Autodesk Inventor part; units mm, degrees
ref_plane "YZ Plane" through (0, 0, 0) normal (1, 0, 0) x (0, 1, 0)
ref_plane "XZ Plane" through (0, 0, 0) normal (0, 1, 0) x (-1, 0, 0)
ref_plane "XY Plane" through (0, 0, 0) normal (0, 0, 1) x (1, 0, 0)
sketch "Sketch1" plane through (0, 0, 0) normal (0, 1, 0) x (-1, 0, 0)
  circle A0 centre (0, 0) radius 13
  line L0 (-10.6616, 0) -> (-8.6254, 6.2667)
  line L1 (-8.6254, 6.2667) -> (-3.2946, 10.1398)
  line L2 (-3.2946, 10.1398) -> (3.2946, 10.1398)
  line L3 (3.2946, 10.1398) -> (8.6254, 6.2667)
  line L4 (8.6254, 6.2667) -> (10.6616, 0)
  line L5 (10.6616, 0) -> (8.6254, -6.2667)
  line L6 (8.6254, -6.2667) -> (3.2946, -10.1398)
  line L7 (3.2946, -10.1398) -> (-3.2946, -10.1398)
  line L8 (-3.2946, -10.1398) -> (-8.6254, -6.2667)
  line L9 (-8.6254, -6.2667) -> (-10.6616, 0)
  line L10 (-11.3, 0) -> (-9.1419, 6.642)
  line L11 (-9.1419, 6.642) -> (-3.4919, 10.7469)
  line L12 (-3.4919, 10.7469) -> (3.4919, 10.7469)
  line L13 (3.4919, 10.7469) -> (9.1419, 6.642)
  line L14 (9.1419, 6.642) -> (11.3, 0)
  line L15 (11.3, 0) -> (9.1419, -6.642)
  line L16 (9.1419, -6.642) -> (3.4919, -10.7469)
  line L17 (3.4919, -10.7469) -> (-3.4919, -10.7469)
  line L18 (-3.4919, -10.7469) -> (-9.1419, -6.642)
  line L19 (-9.1419, -6.642) -> (-11.3, 0)
  circle A1 centre (-6, 0) radius 3.75
  circle A2 centre (6, 0) radius 3.75
  line L20 (9.4432, -3.75) -> (-9.4432, -3.75)
  line L21 (-9.4432, 3.75) -> (9.4432, 3.75)
  dimension "d0" = 26
  dimension "d8" = 7.5
  dimension "d9" = 7.5
extrude "Extrusion1" add sketch "Sketch1" against normal blind 3 contours L10 L11 L12 L13 L14 L15 L16 L17 L18 L19
extrude "Extrusion2" add sketch "Sketch1" along normal blind 20 contours A0
extrude "Extrusion3" add sketch "Sketch1" along normal blind 15 contours L0 L1 L2 L3 L4 L21 | L20 L5 L6 L7 L8 L9 | L10 L11 L12 L13 L14 L15 L16 L17 L18 L19
properties part number "Probe P2"
Could you check a few things on this model? Use its own coordinates, in mm. A direction names the side the tool comes from. Give positions to 0.01 mm unless a question says otherwise; leave off trailing zeros. Order: outer loops, then holes, each group sorted by start corner. A loop starts at its lowest first (then second) coordinate and runs counter-clockwise, first axis right, second up. Notation, with made-up numbers: (67, 24.5) -> (122, 24.5) arc R13 ccw to (122, 43.5) -> close; hole circle Ø3 at (85, 1). An arc over 180 degrees is marked (long way). Answer in a Markdown table with one row per item. Add a question column.
Item 1: Imagine slicing it at D-D (z = -4.75). List the corners of the cut face in (x, y) for me, and give its area (3 significant figures).
Item 2: Imagine slicing it at C-C (y = -0.5). List the corners of the cut face in (x, z) for me, and give its area (3 significant figures).
Item 3: Please list where these lines run through material, in increasing order: probe 1 along Z at (x, y) = (-1.25, -0.75); probe 2 along Y at (x, z) = (-7, 6); probe 3 along X at (y, z) = (14.25, -1.5).
Item 4: I'm going to push flat-ended pins straight in: P1, Ø10, axis at x = 2, z = -2.5, coming from the -Y side; P2, Ø1, axis at y = 14.5, z = 8, coming from the +X side; P3, Ø1, axis at x = -2, y = 15.5, coming from the -Z side. Where does each tip first touch, or does it pass through?
Item 5: We'd pull the mould along X, two halves only. Please class faces 4 (the flat face through (-7, -3, -8)), 5 (the cylindrical face through (10.316, 9.86, 7.91)), 6 (the flat face through (10.236, 17.465, 3.275)), 7 (the flat face through (-6.356, -1.479, -8.666)): pulls with the +X half, pulls with the -X half, needs draft (parallel to the pull), parting line crosses it, or undercut.
Item 6: Imagine slicing it at B-B (z = 0.5). List the corners of the cut face in (x, y) for me, and give its area (3 significant figures).
Item 7: Imagine slicing it at A-A (x = 0). List the corners of the cut face in (y, z) for me.
Item 8: For faces 1 (the flat face through (-10.236, 17.465, -3.275)), 2 (the flat face through (6.28, -1.48, -8.72)), 3 (the flat face through (-5.997, -1.479, -8.176)), which set-ups out of +Z, -Z, +X, -X, +Y, -Y let a thin tool reach every point of the face, with its end or its side?
Result:
| question | item | result |
|---|---|---|
| 1 | outline | (-12.1, 0) -> (-9.76, 0) -> (-9.76, -3) -> (-9.12, -3) -> (-9.12, 0) -> (9.12, 0) -> (9.12, -3) -> (9.76, -3) -> (9.76, 0) -> (12.1, 0) -> (12.1, 20) -> (9.76, 20) -> (9.76, 15) -> (-9.76, 15) -> (-9.76, 20) -> (-12.1, 20) -> close |
| 1 | area | 390 mm2 |
| 2 | outline | (-11.3, 0) -> (-9.14, -6.64) -> (-3.49, -10.75) -> (3.49, -10.75) -> (9.14, -6.64) -> (11.3, 0) -> (9.14, 6.64) -> (3.49, 10.75) -> (-3.49, 10.75) -> (-9.14, 6.64) -> close; hole (-10.66, 0) -> (-8.63, -6.27) -> (-3.29, -10.14) -> (3.29, -10.14) -> (8.63, -6.27) -> (10.66, 0) -> (8.63, 6.27) -> (3.29, 10.14) -> (-3.29, 10.14) -> (-8.63, 6.27) -> close |
| 2 | area | 41.2 mm2 |
| 3 | probe 1 | -10.75 to -10.14, 10.14 to 10.75 |
| 3 | probe 2 | 0 to 15 |
| 3 | probe 3 | -12.91 to -10.17, 10.17 to 12.91 |
| 4 | P1 | y = 0 |
| 4 | P2 | x = 10.62 |
| 4 | P3 | z = -12.91 |
| 5 | face 4 | needs draft |
| 5 | face 5 | parting line crosses it |
| 5 | face 6 | undercut |
| 5 | face 7 | pulls with the -X half |
| 6 | outline | (-12.99, 0) -> (-11.14, 0) -> (-11.14, -3) -> (-10.5, -3) -> (-10.5, 15) -> (-11.14, 15) -> (-11.14, 20) -> (-12.99, 20) -> close; (10.5, -3) -> (11.14, -3) -> (11.14, 0) -> (12.99, 0) -> (12.99, 20) -> (11.14, 20) -> (11.14, 15) -> (10.5, 15) -> close |
| 6 | area | 97.1 mm2 |
| 7 | outline | (-3, -10.75) -> (0, -10.75) -> (0, -13) -> (20, -13) -> (20, -10.75) -> (15, -10.75) -> (15, -3.75) -> (0, -3.75) -> (0, -10.14) -> (-3, -10.14) -> close; (-3, 10.14) -> (0, 10.14) -> (0, 3.75) -> (15, 3.75) -> (15, 10.75) -> (20, 10.75) -> (20, 13) -> (0, 13) -> (0, 10.75) -> (-3, 10.75) -> close |
| 8 | face 1 | +Y |
| 8 | face 2 | -Z, +X, -Y |
| 8 | face 3 | -Y |
